from build123d import *

# Parameters (mm, degrees)
F0_R     = 74.7300726791
F0_W     = 2.6575055344
F0_H     = 17.5374883535
F0_H_2   = 24.9006732447
F2_DEPTH = 25.4
F1_W     = 46.1440682411
F1_H     = 48.5022477806
F3_DEPTH = 41.148


with BuildPart() as f2:
    # F0 (on Front) → F2 (new body)
    with BuildSketch(Plane.XZ):
        Circle(F0_R)
        with BuildLine():
            add(Edge.make_bspline(
                [(-47.0298489993, 22.4099815138), (-44.0062323942, 19.3863649086), (-44.0062323942, 13.9587042795)],
                knots=[0, 0, 0, 1, 1, 1], degree=2))
            add(Edge.make_bspline(
                [(-44.0062323942, 13.9587042795), (-44.0062323942, 8.1674927969), (-47.1501792114, 5.1029127153)],
                knots=[0, 0, 0, 1, 1, 1], degree=2))
            add(Edge.make_bspline(
                [(-47.1501792114, 5.1029127153), (-50.2941260287, 2.0383326337), (-56.1979870715, 2.0383326337)],
                knots=[0, 0, 0, 1, 1, 1], degree=2))
            Line((-56.1979870715, 2.0383326337), (-62.6804572191, 2.0383326337))
            Line((-62.6804572191, 2.0383326337), (-62.6804572191, 25.433598119))
            Line((-62.6804572191, 25.433598119), (-55.511848841, 25.433598119))
            add(Edge.make_bspline(
                [(-55.511848841, 25.433598119), (-50.0534656045, 25.433598119), (-47.0298489993, 22.4099815138)],
                knots=[0, 0, 0, 1, 1, 1], degree=2))
        make_face(mode=Mode.SUBTRACT)
        with BuildLine():
            Line((-26.4329009988, 2.0383326337), (-28.4042683027, 2.0383326337))
            Line((-28.4042683027, 2.0383326337), (-28.931673062, 4.5371046969))
            Line((-28.931673062, 4.5371046969), (-29.0596839259, 4.5371046969))
            add(Edge.make_bspline(
                [(-29.0596839259, 4.5371046969), (-30.3705151722, 2.8883247699), (-31.6736657666, 2.3020350133)],
                knots=[0, 0, 0, 1, 1, 1], degree=2))
            add(Edge.make_bspline(
                [(-31.6736657666, 2.3020350133), (-32.976816361, 1.7157452567), (-34.9328223613, 1.7157452567)],
                knots=[0, 0, 0, 1, 1, 1], degree=2))
            add(Edge.make_bspline(
                [(-34.9328223613, 1.7157452567), (-37.5391235502, 1.7157452567), (-39.0189291368, 3.0624195448)],
                knots=[0, 0, 0, 1, 1, 1], degree=2))
            add(Edge.make_bspline(
                [(-39.0189291368, 3.0624195448), (-40.4987347235, 4.409093833), (-40.4987347235, 6.887384158)],
                knots=[0, 0, 0, 1, 1, 1], degree=2))
            add(Edge.make_bspline(
                [(-40.4987347235, 6.887384158), (-40.4987347235, 12.1972747923), (-32.0039337954, 12.4532965201)],
                knots=[0, 0, 0, 1, 1, 1], degree=2))
            Line((-32.0039337954, 12.4532965201), (-29.0289613185, 12.5505847767))
            Line((-29.0289613185, 12.5505847767), (-29.0289613185, 13.641237337))
            add(Edge.make_bspline(
                [(-29.0289613185, 13.641237337), (-29.0289613185, 15.704772463), (-29.9147964967, 16.6878958977)],
                knots=[0, 0, 0, 1, 1, 1], degree=2))
            add(Edge.make_bspline(
                [(-29.9147964967, 16.6878958977), (-30.8006316748, 17.6710193324), (-32.7566376751, 17.6710193324)],
                knots=[0, 0, 0, 1, 1, 1], degree=2))
            add(Edge.make_bspline(
                [(-32.7566376751, 17.6710193324), (-34.948183665, 17.6710193324), (-37.7132183251, 16.3294654788)],
                knots=[0, 0, 0, 1, 1, 1], degree=2))
            Line((-37.7132183251, 16.3294654788), (-38.5324878541, 18.3622779975))
            add(Edge.make_bspline(
                [(-38.5324878541, 18.3622779975), (-37.2370179114, 19.0637775316), (-35.6932068929, 19.463171427)],
                knots=[0, 0, 0, 1, 1, 1], degree=2))
            add(Edge.make_bspline(
                [(-35.6932068929, 19.463171427), (-34.1493958743, 19.8625653223), (-32.5927837694, 19.8625653223)],
                knots=[0, 0, 0, 1, 1, 1], degree=2))
            add(Edge.make_bspline(
                [(-32.5927837694, 19.8625653223), (-29.4590778212, 19.8625653223), (-27.94598941, 18.4723673404)],
                knots=[0, 0, 0, 1, 1, 1], degree=2))
            add(Edge.make_bspline(
                [(-27.94598941, 18.4723673404), (-26.4329009988, 17.0821693585), (-26.4329009988, 14.0099086251)],
                knots=[0, 0, 0, 1, 1, 1], degree=2))
            Line((-26.4329009988, 14.0099086251), (-26.4329009988, 2.0383326337))
        make_face(mode=Mode.SUBTRACT)
        with BuildLine():
            Line((-6.30447276, 2.0383326337), (-8.9619782945, 2.0383326337))
            Line((-8.9619782945, 2.0383326337), (-8.9619782945, 13.3852156093))
            add(Edge.make_bspline(
                [(-8.9619782945, 13.3852156093), (-8.9619782945, 15.5255572536), (-9.9374210774, 16.5829269893)],
                knots=[0, 0, 0, 1, 1, 1], degree=2))
            add(Edge.make_bspline(
                [(-9.9374210774, 16.5829269893), (-10.9128638602, 17.6402967251), (-12.9968807244, 17.6402967251)],
                knots=[0, 0, 0, 1, 1, 1], degree=2))
            add(Edge.make_bspline(
                [(-12.9968807244, 17.6402967251), (-15.7465540809, 17.6402967251), (-17.0266627198, 16.1528104866)],
                knots=[0, 0, 0, 1, 1, 1], degree=2))
            add(Edge.make_bspline(
                [(-17.0266627198, 16.1528104866), (-18.3067713588, 14.6653242482), (-18.3067713588, 11.2397535304)],
                knots=[0, 0, 0, 1, 1, 1], degree=2))
            Line((-18.3067713588, 11.2397535304), (-18.3067713588, 2.0383326337))
            Line((-18.3067713588, 2.0383326337), (-20.9642768932, 2.0383326337))
            Line((-20.9642768932, 2.0383326337), (-20.9642768932, 19.5758209872))
            Line((-20.9642768932, 19.5758209872), (-18.8034535107, 19.5758209872))
            Line((-18.8034535107, 19.5758209872), (-18.373337008, 17.1743371805))
            Line((-18.373337008, 17.1743371805), (-18.2453261441, 17.1743371805))
            add(Edge.make_bspline(
                [(-18.2453261441, 17.1743371805), (-17.4260566152, 18.4698071231), (-15.9539316804, 19.1841077437)],
                knots=[0, 0, 0, 1, 1, 1], degree=2))
            add(Edge.make_bspline(
                [(-15.9539316804, 19.1841077437), (-14.4818067456, 19.8984083642), (-12.6742933474, 19.8984083642)],
                knots=[0, 0, 0, 1, 1, 1], degree=2))
            add(Edge.make_bspline(
                [(-12.6742933474, 19.8984083642), (-9.5047443574, 19.8984083642), (-7.9046085587, 18.3699586493)],
                knots=[0, 0, 0, 1, 1, 1], degree=2))
            add(Edge.make_bspline(
                [(-7.9046085587, 18.3699586493), (-6.30447276, 16.8415089344), (-6.30447276, 13.4773834313)],
                knots=[0, 0, 0, 1, 1, 1], degree=2))
            Line((-6.30447276, 13.4773834313), (-6.30447276, 2.0383326337))
        make_face(mode=Mode.SUBTRACT)
        with Locations((0.4775428091, 10.8070768104)):
            Rectangle(F0_W, F0_H, mode=Mode.SUBTRACT)
        with BuildLine():
            add(Edge.make_bspline(
                [(17.8793396468, 1.9820078536), (16.6248331807, 1.7157452567), (14.8480423898, 1.7157452567)],
                knots=[0, 0, 0, 1, 1, 1], degree=2))
            add(Edge.make_bspline(
                [(14.8480423898, 1.7157452567), (10.961632562, 1.7157452567), (8.7112015747, 4.086506456)],
                knots=[0, 0, 0, 1, 1, 1], degree=2))
            add(Edge.make_bspline(
                [(8.7112015747, 4.086506456), (6.4607705875, 6.4572676553), (6.4607705875, 10.6611444256)],
                knots=[0, 0, 0, 1, 1, 1], degree=2))
            add(Edge.make_bspline(
                [(6.4607705875, 10.6611444256), (6.4607705875, 14.9059846723), (8.5499078862, 17.4021965183)],
                knots=[0, 0, 0, 1, 1, 1], degree=2))
            add(Edge.make_bspline(
                [(8.5499078862, 17.4021965183), (10.639045185, 19.8984083642), (14.1619041594, 19.8984083642)],
                knots=[0, 0, 0, 1, 1, 1], degree=2))
            add(Edge.make_bspline(
                [(14.1619041594, 19.8984083642), (17.4543435787, 19.8984083642), (19.3745065371, 17.7299043298)],
                knots=[0, 0, 0, 1, 1, 1], degree=2))
            add(Edge.make_bspline(
                [(19.3745065371, 17.7299043298), (21.2946694955, 15.5614002955), (21.2946694955, 12.0078187138)],
                knots=[0, 0, 0, 1, 1, 1], degree=2))
            Line((21.2946694955, 12.0078187138), (21.2946694955, 10.3283161795))
            Line((21.2946694955, 10.3283161795), (9.2155643785, 10.3283161795))
            add(Edge.make_bspline(
                [(9.2155643785, 10.3283161795), (9.2974913314, 7.2406941423), (10.777296918, 5.6405583437)],
                knots=[0, 0, 0, 1, 1, 1], degree=2))
            add(Edge.make_bspline(
                [(10.777296918, 5.6405583437), (12.2571025046, 4.040422545), (14.9453306464, 4.040422545)],
                knots=[0, 0, 0, 1, 1, 1], degree=2))
            add(Edge.make_bspline(
                [(14.9453306464, 4.040422545), (17.7769309557, 4.040422545), (20.5419656158, 5.2232429274)],
                knots=[0, 0, 0, 1, 1, 1], degree=2))
            Line((20.5419656158, 5.2232429274), (20.5419656158, 2.852481728))
            add(Edge.make_bspline(
                [(20.5419656158, 2.852481728), (19.133846113, 2.2482704505), (17.8793396468, 1.9820078536)],
                knots=[0, 0, 0, 1, 1, 1], degree=2))
        make_face(mode=Mode.SUBTRACT)
        with Locations((27.1550068446, 14.488669256)):
            Rectangle(F0_W, F0_H_2, mode=Mode.SUBTRACT)
        with BuildLine():
            add(Edge.make_bspline(
                [(-0.628471055, 22.9911508359), (-1.0765090786, 23.4315082077), (-1.0765090786, 24.3275842549)],
                knots=[0, 0, 0, 1, 1, 1], degree=2))
            add(Edge.make_bspline(
                [(-1.0765090786, 24.3275842549), (-1.0765090786, 25.2390216059), (-0.628471055, 25.664017674)],
                knots=[0, 0, 0, 1, 1, 1], degree=2))
            add(Edge.make_bspline(
                [(-0.628471055, 25.664017674), (-0.1804330313, 26.0890137421), (0.49546433, 26.0890137421)],
                knots=[0, 0, 0, 1, 1, 1], degree=2))
            add(Edge.make_bspline(
                [(0.49546433, 26.0890137421), (1.1355186495, 26.0890137421), (1.5989179768, 25.6563370222)],
                knots=[0, 0, 0, 1, 1, 1], degree=2))
            add(Edge.make_bspline(
                [(1.5989179768, 25.6563370222), (2.0623173041, 25.2236603022), (2.0623173041, 24.3275842549)],
                knots=[0, 0, 0, 1, 1, 1], degree=2))
            add(Edge.make_bspline(
                [(2.0623173041, 24.3275842549), (2.0623173041, 23.4315082077), (1.5989179768, 22.9911508359)],
                knots=[0, 0, 0, 1, 1, 1], degree=2))
            add(Edge.make_bspline(
                [(1.5989179768, 22.9911508359), (1.1355186495, 22.5507934641), (0.49546433, 22.5507934641)],
                knots=[0, 0, 0, 1, 1, 1], degree=2))
            add(Edge.make_bspline(
                [(0.49546433, 22.5507934641), (-0.1804330313, 22.5507934641), (-0.628471055, 22.9911508359)],
                knots=[0, 0, 0, 1, 1, 1], degree=2))
        make_face(mode=Mode.SUBTRACT)
        Polygon((60.7937016587, 25.433598119), (60.7937016587, 2.0383326337), (58.0747509096, 2.0383326337), (58.0747509096, 13.0472669286), (45.7498649339, 13.0472669286), (45.7498649339, 2.0383326337), (43.0309141848, 2.0383326337), (43.0309141848, 25.433598119), (45.7498649339, 25.433598119), (45.7498649339, 15.4794733426), (58.0747509096, 15.4794733426), (58.0747509096, 25.433598119), align=None, mode=Mode.SUBTRACT)
    extrude(amount=F2_DEPTH)

    # F1 (on face) → F3 (join)
    with BuildSketch(Plane.XZ):
        with Locations((-2.2770911455, -36.7938820273)):
            Rectangle(F1_W, F1_H)
    extrude(amount=-F3_DEPTH)


solid = f2.part
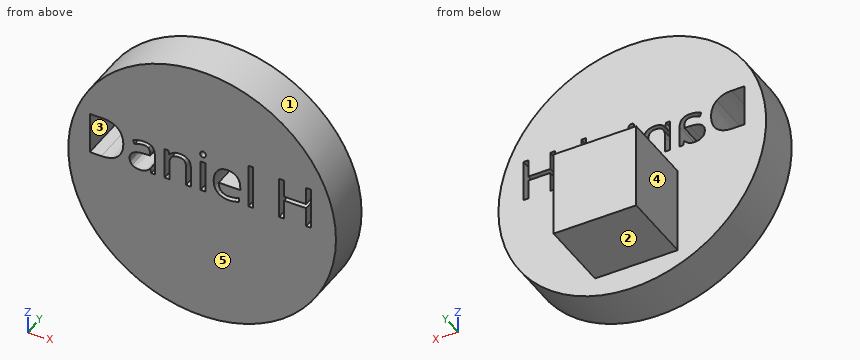
Input: part model. Units: mm. Frame: model coordinates. Face numbers are marked on the shaded views. A direction names the side the tool comes from. Give positions to 0.01 mm unless a question says otherwise; leave off trailing zeros. Loops run counter-clockwise (first coordinate to the right, second up) from the corner with the lowest first, then second, coordinate; pieces in that order, holes last. Notation, with made-up numbers: M 4,-27.75 L 21,-27.75 A14 cw 21,-19.75 Z; hole C 22.25,-27.5 d5. An arc over 180 degrees is marked long. Use CSV: the item, a comma, the result in double quotes.
(1) Set-up query: the marked faces 1 and 2. Return all of +Z, -Z, +X, -X, +Y, -Y with unobstructed straight access to the full face (end or side cutting, diameter ignored); none if empty.
Outcome:
face 1,"+Y, -Y"
face 2,"-Z, +X, -X, +Y"
(2) Pull-direction query (X, two-part tool) for the marked faces 3, 4 and 5; classes: pulls with the +X half, pulls with the -X half, needs draft (parallel to the pull), parting line crosses it, or undercut.
Outcome:
face 3,"undercut"
face 4,"pulls with the -X half"
face 5,"needs draft"
(3) Pin query (flat end, axial travel): P1, Ø1.3, axis at x = 1, y = -14.5, coming from the +Z side; P2, Ø6, axis at x = 4, z = 24, coming from the +Y side; P3, Ø11.5, axis at y = -17, z = 16, coming from the +X side. Return the tip coordinate at first contact, or that it passes through.
Outcome:
P1,"stops at z = 74.73"
P2,"stops at y = 0"
P3,"stops at x = 74.02"
(4) Section B-B, the plane y = -8.5. Count the separate pieces of the cut face and the enclosed holes in it, plus the area to 3 significant figures.
Outcome:
separate pieces,"1"
enclosed holes,"8"
area,"16,400 mm²"
(5) Section C-C, the plane z = -46. Return loops of the section in (x, y), plus the area to 3 significant figures.
Outcome:
outline,"M -58.89,-25.4 L 58.89,-25.4 L 58.89,0 L 20.79,0 L 20.79,41.15 L -25.35,41.15 L -25.35,0 L -58.89,0 Z"
area,"4,890 mm²"
(6) Section D-D, the plane y = 6.5. Return loops of the section in (x, z) (3 decimals).
Outcome:
outline,"M -25.349,-61.045 L 20.795,-61.045 L 20.795,-12.543 L -25.349,-12.543 Z"
(7) Material intervals for L1, parallel to Y at x = 41.5, z = -42.5; L2, parallel to Z at x = 5.5, y = 13 (3 decimals); L3, parallel to Z at x = 10, y = -8.5, sorted ascending. Write a range as [from, to].
Outcome:
L1,"y = [-25.4, 0]"
L2,"z = [-61.045, -12.543]"
L3,"z = [-74.06, 3.01], [6.76, 10.33], [18.72, 74.06]"
(8) Section A-A, the plane x = 4.5. Return loops of the section in (y, z) (3 decimals), plus the area to 3 significant figures.
Outcome:
outline,"M -25.4,-74.594 L 0,-74.594 L 0,-61.045 L 41.148,-61.045 L 41.148,-12.543 L 0,-12.543 L 0,74.594 L -25.4,74.594 Z"
area,"5,790 mm²"
